Part model, mm, in its own coordinate system. A direction names the side the tool comes from. Coordinates: 2 decimals unless noted, no trailing zeros. Answer as a JSON object with one key per item and string values. Group by question number.
1. Drill centre lines: L1, parallel to Y at x = -4.3, z = -20; L2, parallel to X at y = -18, z = 15; L3, parallel to Z at x = -3.25, y = 18. Where is each one in solid material? Low to high.
2. Drop flat-ended pins along their axis: pin 1 Ø15.5 at (y, z) = (-10, 5.5) entering from -X; pin 2 Ø5 at (y, z) = (-15.5, -35.5) entering from +X; pin 3 Ø1.2 at (x, z) = (-3, -48) entering from +Y; pin 4 Ø7 at (y, z) = (25.5, -8) entering from -X. Give the stop position or say it passes through.
3. Saw through at A-A on z = 0.5. Count the separate pieces of the cut face and the enclosed holes in it, then the cut area to 3 significant figures.
4. 3-axis set-ups, long thin cutter, end or side, ignore diameter. For faces 4 (the face through (-3.75, 2, 5)), 5 (the face through (-1.25, -25, -18)), 6 (the face through (-2.48, 19.33, -31.16)): which of +Z, -Z, +X, -X, +Y, -Y reach the whole face in a straight line?
5. Mould opens along Y. For faces 1 (the face through (-3.75, -8.7, -58.3)), 2 (the face through (-4.38, -39.05, -28.67)), 3 (the face through (-3.75, 22, -9)) say: released by +Y, released by -Y, zero draft, split by the parting line, or undercut.
from build123d import *
from build123d import SkipClean  # not in build123d's __all__

# Parameters (mm, degrees)
F3_DEPTH        = 2.5
F3_COPIES_COUNT = 12


# Not quite as in the source:
# - after a boolean that leaves OpenCascade's solid faulty, fix() repairs it
# - a pattern or mirror of a feature is missing from the dataset's text; its kind, count and spacing are read off the source's solid


with BuildPart() as f1:
    # F0 (on Front) → F1 (revolve)
    with BuildSketch(Plane.XZ):
        Polygon((-5, -20), (0, -20), (0, -10), (-1.25, -10), (-1.25, 15), (0, 15), (0, 20), (-1.25, 20), (-1.25, 19), (-3.75, 19), (-3.75, 20), (-5, 20), (-5, 15), (-3.75, 15), (-3.75, -10), (-5, -10), align=None)
    revolve(axis=Axis((-2.5, 0, -20), (-1, 0, 0)))

    # F2 (on face) → F3 (cut, through all)
    with BuildSketch(Plane.YZ.offset(-1.25)):
        with BuildLine():
            Line((0, -10), (0, 15))
            ThreePointArc((0, 15), (-6.1307239653, 14.4588772838), (-12.0718779875, 12.8522413521))
            Line((-12.0718779875, 12.8522413521), (-3.1961564517, -10.5245272447))
            ThreePointArc((-3.1961564517, -10.5245272447), (-1.6194555331, -10.1320030515), (0, -10))
        make_face()
    with SkipClean():  # cleaning this boolean's faces spoils the solid; the shape is the same uncleaned
        f3 = extrude(amount=-F3_DEPTH, mode=Mode.SUBTRACT)

    # F3_copies: F3 ×12 about axis
    f3_copies_axis = Axis((0, 0, -20), (1, 0, 0))
    for i in range(1, F3_COPIES_COUNT):
        add(f3.rotate(f3_copies_axis, i * 360 / F3_COPIES_COUNT), clean=False, mode=Mode.SUBTRACT)

    add(f1.part.fix(), mode=Mode.REPLACE)


solid = f1.part
Outcome:
{
 "1": {"L1": "y = -40 to -35, -10 to 10, 35 to 40", "L2": "x = -5 to -3.75, -1.25 to 0", "L3": "z = -54.6 to -50.02, -35.17 to -30.39, -23.3 to -20, -13.57 to -9.61, 1.47 to 14.6"},
 "2": {"pin 1": "stops at x = -5", "pin 2": "stops at x = -1.25", "pin 3": "stops at y = 27.75", "pin 4": "stops at x = -3.75"},
 "3": {"separate pieces": "5", "enclosed holes": "0", "area": "97.4 mm²"},
 "4": {"face 4": "-X", "face 5": "+X", "face 6": "+X, -X"},
 "5": {"face 1": "zero draft", "face 2": "split by the parting line", "face 3": "undercut"}
}
